from build123d import *

# Parameters (mm, degrees)
BOSS_EXTRUDE1_DEPTH      = 15
BOSS_EXTRUDE1_DEPTH_BACK = 15
SKETCH2_W                = 10.45
SKETCH2_H                = 4
CUT_EXTRUDE3_DEPTH       = 28.414640249
CUT_EXTRUDE7_DEPTH       = 5
CHAMFER1_SIZE            = 1.5
CHAMFER2_SIZE            = 0.5
CHAMFER2_SIZE2           = 1.104400541
CHAMFER2_EDGE_2_SIZE     = 0.5
CHAMFER2_EDGE_2_SIZE2    = 1.104400541


with BuildPart() as part:
    # Sketch1 → Boss-Extrude1 (new, two sides)
    with BuildSketch(Plane.XY) as boss_extrude1_sk:
        Polygon((20, 5), (20, 0), (0, 0), (0, 12.25), (-5.154982838, 12.25), (-5.154982838, 16.25), (14.432786844, 16.25), align=None)
    extrude(amount=BOSS_EXTRUDE1_DEPTH)
    extrude(boss_extrude1_sk.sketch, amount=-BOSS_EXTRUDE1_DEPTH_BACK)

    # Sketch2 → Cut-Revolve2 (revolve, cut)
    with BuildSketch(Plane.XY):
        with Locations((5.225, 10.25)):
            Rectangle(SKETCH2_W, SKETCH2_H)
        Polygon((-1.55, 16.25), (-5.154982838, 16.25), (-5.154982838, 12.25), (0, 12.25), (3.45, 12.25), (3.45, 13.85), (-1.55, 15.25), align=None)
    revolve(axis=Axis((-123.55, 0, 0), (0, 1, 0)), mode=Mode.SUBTRACT)

    # Sketch5 → Cut-Extrude3 (cut, through all)
    with BuildSketch(Plane(origin=(0, 5, 0), x_dir=(-1, 0, 0), z_dir=(0, -1, 0))):
        with BuildLine():
            Line((-20, -5.65), (-10, -5.65))
            ThreePointArc((-10, -5.65), (-4.35, 0), (-10, 5.65))
            Line((-10, 5.65), (-20, 5.65))
            Line((-20, 5.65), (-20, -5.65))
        make_face()
    extrude(amount=-CUT_EXTRUDE3_DEPTH, mode=Mode.SUBTRACT)

    # Sketch6 → Cut-Extrude7 (cut)
    with BuildSketch(Plane(origin=(0, 5, 0), x_dir=(1, 0, 0), z_dir=(0, 1, 0))):
        with BuildLine():
            Line((10, 2.9), (14.5, 2.9))
            ThreePointArc((14.5, 2.9), (17.4, 0), (14.5, -2.9))
            Line((14.5, -2.9), (10, -2.9))
            ThreePointArc((10, -2.9), (7.1, 0), (10, 2.9))
        make_face()
    extrude(amount=-CUT_EXTRUDE7_DEPTH, mode=Mode.SUBTRACT)

    # Chamfer1
    chamfer1_edges = [part.edges().sort_by_distance(p)[0] for p in [
        (17.216393422, 10.625, 15),
        (12.216393422, 16.25, -5.65),
        (12.216393422, 16.25, 5.65),
        (17.216393422, 10.625, 5.65),
        (17.216393422, 10.625, -5.65),
        (4.35, 16.25, 0),
        (17.216393422, 10.625, -15),
    ]]
    chamfer(chamfer1_edges, length=CHAMFER1_SIZE)

    # Chamfer2
    chamfer2_edges = [part.edges().sort_by_distance(p)[0] for p in [
        (14.432786844, 16.25, -10.325),
    ]]
    chamfer2_side = [part.faces().sort_by_distance(p)[0] for p in [
        (5.141762366, 16.25, -14.655631739),
    ]]
    chamfer(chamfer2_edges, length=CHAMFER2_SIZE, length2=CHAMFER2_SIZE2, reference=chamfer2_side[0])

    # Chamfer2 edge 2
    chamfer2_edge_2_edges = [part.edges().sort_by_distance(p)[0] for p in [
        (14.432786844, 16.25, 10.325),
    ]]
    chamfer2_edge_2_side = [part.faces().sort_by_distance(p)[0] for p in [
        (5.141762366, 16.25, -14.655631739),
    ]]
    chamfer(chamfer2_edge_2_edges, length=CHAMFER2_EDGE_2_SIZE, length2=CHAMFER2_EDGE_2_SIZE2, reference=chamfer2_edge_2_side[0])


solid = part.part
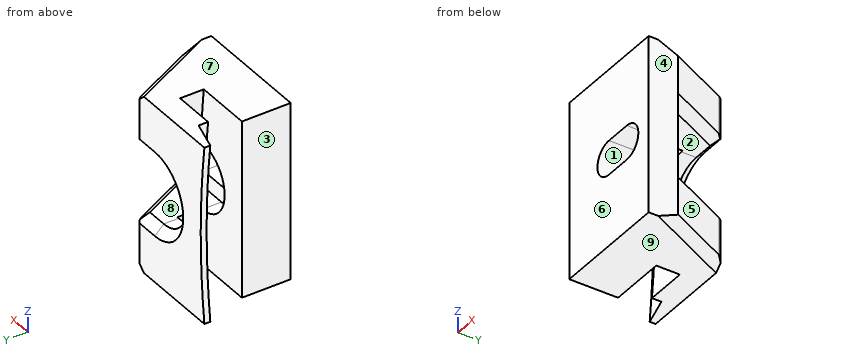
CAD build for the part. Positions are in the model's coordinates, mm. Face numbers are marked on the shaded views. A direction names the side the tool comes from. Give positions to 0.01 mm unless a question says otherwise; leave off trailing zeros. Write each loop counter-clockwise with the first axis right and the second up, starting at its lowest first coordinate (ties: lowest second). Pieces come first, ordered by that corner, then holes. Notation, with made-up numbers: M 25.25,43.25 L 50.25,43.25 A23 ccw 50.25,66.25 Z; hole C 47.25,60.5 d11. An arc over 180 degrees is marked long. Put each result on its own line as item: value. Start each with the question number.
(1) Band-saw the part on B-B, the plane y = 10. Write the cut outline in (x, z), and give its area (3 significant figures).
(2) Band-saw the part on D-D, the plane y = 7.5. Write the cut outline in (x, z).
(3) Band-saw the part on A-A, the plane z = 0. Write the cut outline in (x, y).
(4) Probe L1, parallel to Z at x = 10.25, y = 0.5; L2, parallel to Z at x = 11, y = 9; L3, parallel to Y at x = 5, z = 6.5. List the from-to ranges inside material, lowest first.
(5) Which spindle directions (+Z, -Z, +X, -X, +Y, -Y) get a long thin tool onto all of the face, cutting with end or side? Do the marked faces 1, 2, 3, 4 and 5. Say none if no direction does.
(6) Flat gauge pins, fed straight in: pin 1 Ø3 at (y, z) = (8, 9.5) entering from +X; pin 2 Ø7 at (x, z) = (16, 1) entering from +Y; pin 3 Ø8 at (y, z) = (5.5, 3) entering from -X. Where does each tip first touch, or does it go through?
(7) Band-saw the part on C-C, the plane y = 3.75. Write the cut outline in (x, z).
(8) Mould opens along Z. For the marked faces 6, 7, 8 and 9 say: +Z half, -Z half, draft (parallel to the pull), parting line (faces both ways), or undercut.
Response values:
1. outline: M 9.61,-15 L 15.85,-15 L 17.53,-13.5 L 17.53,-7.15 L 15.85,-5.65 L 10.33,-5.65 A134 cw Z; M 9.61,15 A134 cw 10.33,5.65 L 15.85,5.65 L 17.53,7.15 L 17.53,13.5 L 15.85,15 Z
1. area: 135 mm2
2. outline: M 0,-15 L 17.09,-15 L 18.76,-13.5 L 18.76,-7.15 L 17.09,-5.65 L 10,-5.65 A5.65 cw 10,5.65 L 17.09,5.65 L 18.76,7.15 L 18.76,13.5 L 17.09,15 L 0,15 Z
3. outline: M -1.55,15.25 L 3.45,13.85 L 3.45,12.25 L 4.35,12.25 L 4.35,14.75 L 2.85,16.25 L -1.55,16.25 Z; M 0,0 L 7.1,0 L 7.1,5 L 4.35,5 L 4.35,8.25 L 0,8.25 Z; M 17.4,0 L 20,0 L 20,5 L 17.4,5 Z
4. L1: z = -15 to -2.9, 2.9 to 15
4. L2: z = -15 to -5.65, 5.65 to 15
4. L3: y = 0 to 8.25, 12.25 to 16.25
5. face 1: +Y, -Y
5. face 2: +X, +Y
5. face 3: +Z, -Z, -X, -Y
5. face 4: +Z, -Z, +X, +Y, -Y
5. face 5: +Z, -Z, +X, +Y
6. pin 1: stops at x = 19.26
6. pin 2: stops at y = 5
6. pin 3: stops at x = 0
7. outline: M 0,-15 L 18.94,-15 L 20,-14.05 L 20,14.05 L 18.94,15 L 0,15 Z; hole M 10,-2.9 L 14.5,-2.9 A2.9 ccw 14.5,2.9 L 10,2.9 A2.9 ccw Z
8. face 6: draft
8. face 7: +Z half
8. face 8: undercut
8. face 9: -Z half
